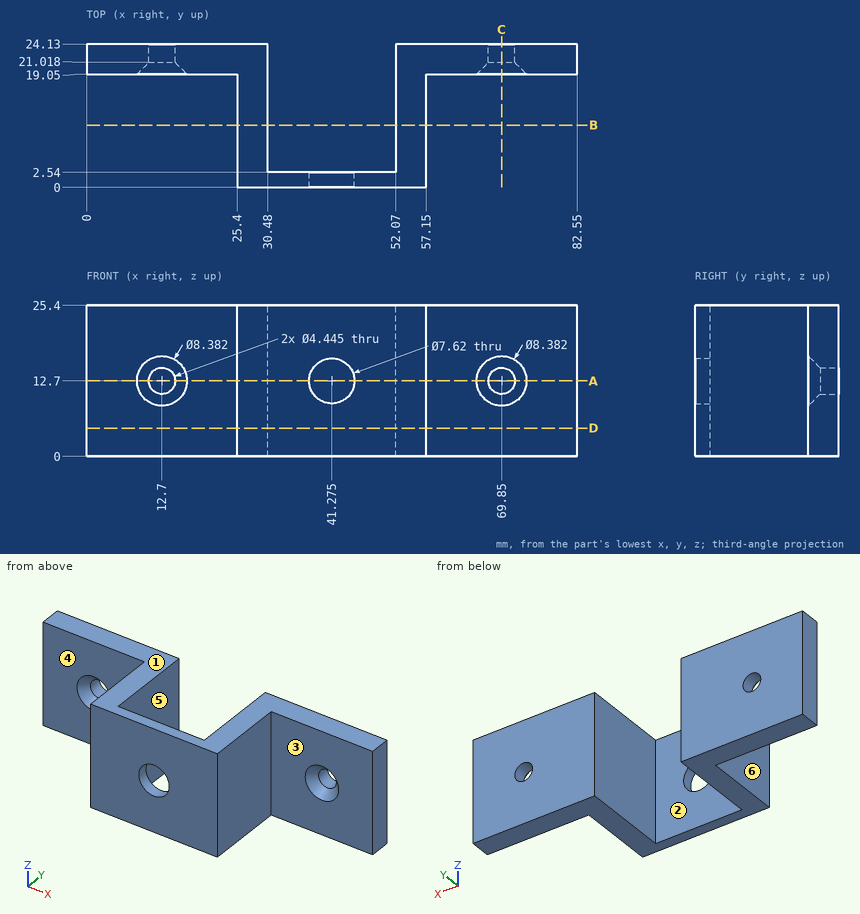
The figure shows three views and two pictorial views of one solid part (mm, origin at its lowest corner). Answer the questions. A direction names the side the tool comes from. Coordinates: 2 decimals unless noted, no trailing zeros. Write each loop counter-clockwise with the first axis right and the second up, starting at its lowest first coordinate (ties: lowest second). Pieces come first, ordered by that corner, then holes.
1. For the marked faces 1, 2 and 3, determine the directions among +Z, -Z, +X, -X, +Y, -Y from which every point of the face is accessible in a straight line to the end or side of a thin tool.
Results list:
face 1: +Z, +X, -X, +Y, -Y
face 2: +Z, -Z, +Y
face 3: +Z, -Z, +X, -Y
2. The part is cut by section A-A, the plane z = 12.7. State how many separate pieces and enclosed holes the cut face has, and give its area (3 significant figures).
Results list:
separate pieces: 4
enclosed holes: 0
area: 486 mm2
3. The part is cut by section D-D, the plane z = 4.75. Write down the section's boundary in (x, y), and give its area (3 significant figures).
Results list:
outline: (0, 19.05) - (25.4, 19.05) - (25.4, 0) - (57.15, 0) - (57.15, 19.05) - (82.55, 19.05) - (82.55, 24.13) - (52.07, 24.13) - (52.07, 2.54) - (30.48, 2.54) - (30.48, 24.13) - (0, 24.13) - close
area: 558 mm2
4. Consider line 1 along Z through (x, y) = (69.85, 22.7); line 2 along X through (y, z) = (2.75, 16.75); line 3 along X through (y, z) = (22.1, 12.7). Determine where each line is inside the solid, lowest interval first.
Results list:
line 1: z = 0 to 10.48, 14.92 to 25.4
line 2: x = 25.4 to 30.48, 52.07 to 57.15
line 3: x = 0 to 10.48, 14.92 to 30.48, 52.07 to 67.63, 72.07 to 82.55
5. The part is cut by section C-C, the plane x = 69.85. Write down the section's boundary in (y, z).
Results list:
outline: (19.05, 0) - (24.13, 0) - (24.13, 10.48) - (21.02, 10.48) - (19.05, 8.51) - close; (19.05, 16.89) - (21.02, 14.92) - (24.13, 14.92) - (24.13, 25.4) - (19.05, 25.4) - close
6. Flat-ended cylindrical pins translate along their axes: pin 1 (12.5 mm diameter, centred on x = 64.5, z = 11.5, fed in from -Y); pin 2 (2 mm diameter, centred on y = 18, z = 4.5, fed in from -X); pin 3 (11 mm diameter, centred on y = 9, z = 10.5, fed in from +X). Find the tip coordinate at first contact, or state that the pin passes through.
Results list:
pin 1: stops at y = 19.05
pin 2: stops at x = 25.4
pin 3: stops at x = 57.15
7. For a pull along X with two mould halves and no side action, classify the marked faces 4, 5 and 6 as +X half, -X half, draft (parallel to the pull), parting line (faces both ways), or undercut.
Results list:
face 4: draft
face 5: undercut
face 6: -X half
8. The part is cut by section B-B, the plane y = 10.5. Write down the section's boundary in (x, z), and give its area (3 significant figures).
Results list:
outline: (25.4, 0) - (30.48, 0) - (30.48, 25.4) - (25.4, 25.4) - close; (52.07, 0) - (57.15, 0) - (57.15, 25.4) - (52.07, 25.4) - close
area: 258 mm2
